```python
from build123d import *

# Parameters (mm, degrees)
EXTRUDE_1_DEPTH     = 4
SKETCH_2_R          = 21.5
CUT_EXTRUDE_1_DEPTH = 5
SKETCH_4_R          = 1.525
CUT_EXTRUDE_3_DEPTH = 5
SKETCH_5_R          = 1.525
CUT_EXTRUDE_4_DEPTH = 5
SKETCH_6_W          = 1
SKETCH_6_H          = 57
EXTRUDE_2_DEPTH     = 4
FILLET_1_R          = 2


with BuildPart() as part:
    # 草图1 → 凸台-拉伸1 (new body)
    with BuildSketch(Plane(origin=(0, 0, 0), x_dir=(1, 0, 0), z_dir=(0, 1, 0))):
        with BuildLine():
            ThreePointArc((19.5, 28.5), (-9, 0), (19.5, -28.5))
            Line((19.5, -28.5), (19.5, 28.5))
        make_face()
        with BuildLine():
            Line((19.5, 28.5), (19.5, -28.5))
            ThreePointArc((19.5, -28.5), (39.652543264, -20.152543264), (48, 0))
            ThreePointArc((48, 0), (39.652543264, 20.152543264), (19.5, 28.5))
        make_face()
        with BuildLine():
            Line((-19.5, 28.5), (-19.5, -28.5))
            Line((-19.5, -28.5), (19.5, -28.5))
            ThreePointArc((19.5, -28.5), (-9, 0), (19.5, 28.5))
            Line((19.5, 28.5), (-19.5, 28.5))
        make_face()
    extrude(amount=EXTRUDE_1_DEPTH)

    # 草图2 → 切除-拉伸1 (cut, through all)
    with BuildSketch(Plane(origin=(0, 4, 0), x_dir=(1, 0, 0), z_dir=(0, 1, 0))):
        with Locations((19.5, 0)):
            Circle(SKETCH_2_R)
    extrude(amount=-CUT_EXTRUDE_1_DEPTH, mode=Mode.SUBTRACT)

    # 草图4 → 切除-拉伸3 (cut, through all)
    with BuildSketch(Plane(origin=(0, 4, 0), x_dir=(1, 0, 0), z_dir=(0, 1, 0))):
        with Locations((-5.5, 0)):
            Circle(SKETCH_4_R)
        with Locations((7, 21.650635095)):
            Circle(SKETCH_4_R)
        with Locations((32, 21.650635095)):
            Circle(SKETCH_4_R)
        with Locations((44.5, 0)):
            Circle(SKETCH_4_R)
        with Locations((32, -21.650635095)):
            Circle(SKETCH_4_R)
        with Locations((7, -21.650635095)):
            Circle(SKETCH_4_R)
    extrude(amount=-CUT_EXTRUDE_3_DEPTH, mode=Mode.SUBTRACT)

    # 草图5 → 切除-拉伸4 (cut, through all)
    with BuildSketch(Plane(origin=(0, 4, 0), x_dir=(1, 0, 0), z_dir=(0, 1, 0))):
        with Locations((-17, 19.5)):
            Circle(SKETCH_5_R)
        with Locations((-17, 0)):
            Circle(SKETCH_5_R)
        with Locations((-17, -19.5)):
            Circle(SKETCH_5_R)
    extrude(amount=-CUT_EXTRUDE_4_DEPTH, mode=Mode.SUBTRACT)

    # 草图6 → 凸台-拉伸2 (add)
    with BuildSketch(Plane(origin=(0, 4, 0), x_dir=(1, 0, 0), z_dir=(0, 1, 0))):
        with Locations((-20, 0)):
            Rectangle(SKETCH_6_W, SKETCH_6_H)
    extrude(amount=-EXTRUDE_2_DEPTH)

    # 圆角1
    fillet_1_edges = [part.edges().sort_by_distance(p)[0] for p in [
        (-20.5, 2, 28.5),
        (-20.5, 2, -28.5),
    ]]
    fillet(fillet_1_edges, radius=FILLET_1_R)


solid = part.part
```
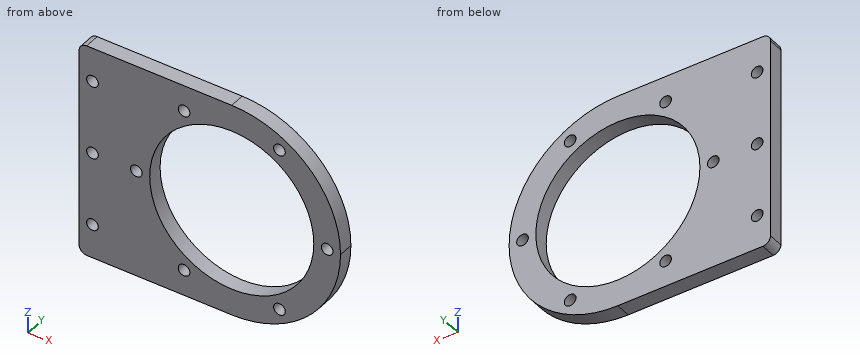
Source: CAD feature listing. Evaluate the final solid. Frame: model axes, mm. Give positions to 0.01 mm unless a question says otherwise; leave off trailing zeros. Loops run counter-clockwise (first coordinate to the right, second up) from the corner with the lowest first, then second, coordinate; pieces in that order, holes last. Notation, with made-up numbers: M 25.25,53 L 38.25,53 A17 ccw 38.25,58 Z; hole C 89,35.25 d4. An arc over 180 degrees is marked long. Put each result on its own line as item: value.
Q1. Section A-A (x = -5.5). Return the cut outline in (y, z) (3 decimals), and give its area (3 significant figures).
Response values:
outline: M 0,-28.5 L 4,-28.5 L 4,-1.525 L 0,-1.525 Z; M 0,1.525 L 4,1.525 L 4,28.5 L 0,28.5 Z
area: 216 mm²
Q2. Section D-D (y = 2.35). Count the separate pieces of the cut face and the enclosed holes in it, and give its area (3 significant figures).
Response values:
separate pieces: 1
enclosed holes: 10
area: 2,040 mm²
Q3. Line query: probe 1 along X at (y, z) = (1.6, 0) (3 decimals); probe 2 along Z at (x, y) = (-17, 1.6) (3 decimals); probe 3 along Z at (x, y) = (-5.5, 2) (3 decimals). Output: solid intervals per line, ascending. Write a range as [from, to].
Response values:
probe 1: x = [-20.5, -18.525], [-15.475, -7.025], [-3.975, -2], [41, 42.975], [46.025, 48]
probe 2: z = [-28.5, -21.025], [-17.975, -1.525], [1.525, 17.975], [21.025, 28.5]
probe 3: z = [-28.5, -1.525], [1.525, 28.5]
Q4. Section C-C (x = -17). Return the cut outline in (y, z) (3 decimals), and give its area (3 significant figures).
Response values:
outline: M 0,-28.5 L 4,-28.5 L 4,-21.025 L 0,-21.025 Z; M 0,-17.975 L 4,-17.975 L 4,-1.525 L 0,-1.525 Z; M 0,1.525 L 4,1.525 L 4,17.975 L 0,17.975 Z; M 0,21.025 L 4,21.025 L 4,28.5 L 0,28.5 Z
area: 191 mm²
Q5. Section B-B (z = -17). Return the cut outline in (x, y).
Response values:
outline: M -20.5,0 L 6.34,0 L 6.34,4 L -20.5,4 Z; M 32.66,0 L 42.37,0 L 42.37,4 L 32.66,4 Z
Q6. Pin query (flat end, axial travel): P1, Ø2.5, axis at x = 7, z = 21.65, coming from the -Y side. Return the tip coordinate at first contact, or that it passes through.
Response values:
P1: passes through
